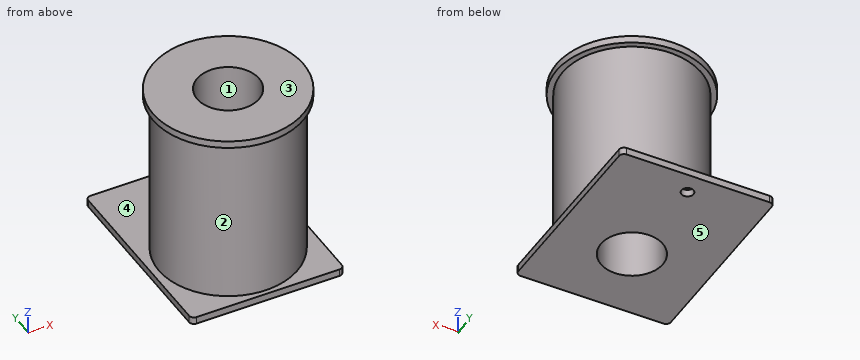
from build123d import *

# Parameters (mm, degrees)
ESQUISSE1_R             = 14.285
BOSS_EXTRU_1_DEPTH      = 35.2
ESQUISSE2_R             = 15.5
BOSS_EXTRU_2_DEPTH      = 1.5
BOSS_EXTRU_3_DEPTH      = 1.5
ESQUISSE3_R             = 6.385
ESQUISSE3_R_2           = 1.25
ENL_V_MAT_EXTRU_1_DEPTH = 39.2


with BuildPart() as part:
    # Esquisse1 → Boss.-Extru.1 (new body)
    with BuildSketch(Plane.XY):
        Circle(ESQUISSE1_R)
    extrude(amount=BOSS_EXTRU_1_DEPTH)

    # Esquisse2 → Boss.-Extru.2 (add)
    with BuildSketch(Plane.XY.offset(35.2)):
        Circle(ESQUISSE2_R)
    extrude(amount=BOSS_EXTRU_2_DEPTH)

    # Esquisse4 → Boss.-Extru.3 (add)
    with BuildSketch(Plane(origin=(0, 0, 0), x_dir=(-1, 0, 0), z_dir=(0, 0, -1))):
        with BuildLine():
            Line((-14.75, 25.285), (14.75, 25.285))
            ThreePointArc((14.75, 25.285), (15.457106781, 24.992106781), (15.75, 24.285))
            Line((15.75, 24.285), (15.75, -14.255))
            ThreePointArc((15.75, -14.255), (15.457106781, -14.962106781), (14.75, -15.255))
            Line((14.75, -15.255), (-14.75, -15.255))
            ThreePointArc((-14.75, -15.255), (-15.457106781, -14.962106781), (-15.75, -14.255))
            Line((-15.75, -14.255), (-15.75, 24.285))
            ThreePointArc((-15.75, 24.285), (-15.457106781, 24.992106781), (-14.75, 25.285))
        make_face()
    extrude(amount=BOSS_EXTRU_3_DEPTH)

    # Esquisse3 → Enlèv. mat.-Extru.1 (cut, through all)
    with BuildSketch(Plane.XY.offset(36.7)):
        Circle(ESQUISSE3_R)
        with Locations((-0.25, 20.785)):
            Circle(ESQUISSE3_R_2)
    extrude(amount=-ENL_V_MAT_EXTRU_1_DEPTH, mode=Mode.SUBTRACT)


solid = part.part
Input: part model. Units: mm. Frame: model coordinates. Face numbers are marked on the shaded views. A direction names the side the tool comes from. Round coordinates to 2 decimals unless told otherwise and drop trailing zeros. Order: outer loops, then holes, each group sorted by start corner. A loop starts at its lowest first (then second) coordinate and runs counter-clockwise, first axis right, second up.
1. Mould query, pull axis X, two halves, no side actions, for the marked faces 1, 2 and 3. Classes: released by +X, released by -X, zero draft, split by the parting line, or undercut.
The answers:
face 1: undercut
face 2: split by the parting line
face 3: zero draft
2. Cut plane D-D, the plane y = 10.5. Output: boundary loops of the cut face in (x, z).
The answers:
outline: (-15.75, -1.5) - (15.75, -1.5) - (15.75, 0) - (9.69, 0) - (9.69, 35.2) - (11.4, 35.2) - (11.4, 36.7) - (-11.4, 36.7) - (-11.4, 35.2) - (-9.69, 35.2) - (-9.69, 0) - (-15.75, 0) - close
3. Pin query (flat end, axial travel): P1, Ø1.2, axis at x = -2.5, z = -1, coming from the -Y side (3 decimals); P2, Ø1, axis at y = -6.5, z = 30, coming from the +X side; P3, Ø1, axis at x = -1.5, y = 18, coming from the +Z side. Return the tip coordinate at first contact, or that it passes through.
The answers:
P1: stops at y = -15.255
P2: stops at x = 12.96
P3: stops at z = 0
4. Material intervals for line 1 (Y direction, x = 0, z = 15) (3 decimals); line 2 (Z direction, x = 4, y = -14); line 3 (Z direction, x = -1, y = 23), sorted ascending.
The answers:
line 1: y = -14.285 to -6.385, 6.385 to 14.285
line 2: z = -1.5 to 0, 35.2 to 36.7
line 3: z = -1.5 to 0
5. Set-up query: the marked faces 4 and 5. Return all of +Z, -Z, +X, -X, +Y, -Y with unobstructed straight access to the full face (end or side cutting, diameter ignored); none if empty.
The answers:
face 4: none
face 5: -Z, +X, -X, +Y, -Y
6. Cut plane A-A, the plane y = 0. Output: boundary loops of the cut face in (x, z) (3 decimals), then the cut area to 3 significant figures.
The answers:
outline: (-15.75, -1.5) - (-6.385, -1.5) - (-6.385, 36.7) - (-15.5, 36.7) - (-15.5, 35.2) - (-14.285, 35.2) - (-14.285, 0) - (-15.75, 0) - close; (6.385, -1.5) - (15.75, -1.5) - (15.75, 0) - (14.285, 0) - (14.285, 35.2) - (15.5, 35.2) - (15.5, 36.7) - (6.385, 36.7) - close
area: 612 mm2
7. Cut plane C-C, the plane x = -9.5. Output: boundary loops of the cut face in (y, z) (3 decimals), then the cut area to 3 significant figures.
The answers:
outline: (-15.255, -1.5) - (25.285, -1.5) - (25.285, 0) - (10.668, 0) - (10.668, 35.2) - (12.247, 35.2) - (12.247, 36.7) - (-12.247, 36.7) - (-12.247, 35.2) - (-10.668, 35.2) - (-10.668, 0) - (-15.255, 0) - close
area: 849 mm2
8. Cut plane B-B, the plane x = -0.25. Output: boundary loops of the cut face in (y, z) (3 decimals).
The answers:
outline: (-15.498, 35.2) - (-14.283, 35.2) - (-14.283, 0) - (-15.255, 0) - (-15.255, -1.5) - (-6.38, -1.5) - (-6.38, 36.7) - (-15.498, 36.7) - close; (6.38, -1.5) - (19.535, -1.5) - (19.535, 0) - (14.283, 0) - (14.283, 35.2) - (15.498, 35.2) - (15.498, 36.7) - (6.38, 36.7) - close; (22.035, -1.5) - (25.285, -1.5) - (25.285, 0) - (22.035, 0) - close
